Could you check a few things on this model? Use its own coordinates, in mm. Face numbers are marked on the shaded views. Give positions to 0.01 mm unless a question says otherwise; leave off trailing zeros. Loops run counter-clockwise (first coordinate to the right, second up) from the corner with the lowest first, then second, coordinate; pieces in that order, holes last. Notation, with made-up numbers: M -21.5,-38.75 L -2.5,-38.75 A27 ccw -2.5,-3.75 Z; hole C 3,-28.5 d5. An arc over 180 degrees is marked long. Use CSV: the item, a comma, the result in double quotes.
```python
from build123d import *

# Parameters (mm, degrees)
SKETCH2_R           = 0.5
BOSS_EXTRUDE1_DEPTH = 3.5


with BuildPart() as part:
    # Sketch1 → Base-Revolve (revolve)
    with BuildSketch(Plane.XY):
        with BuildLine():
            Line((-3.81, 0.1), (1.69, 0.1))
            Line((1.69, 0.1), (1.69, 0))
            Line((1.69, 0), (3.19, 0))
            ThreePointArc((3.19, 0), (3.897106781, 0.292893219), (4.19, 1))
            Line((4.19, 1), (4.19, 1.21))
            ThreePointArc((4.19, 1.21), (4.049208002, 2.388175538), (3.634760961, 3.5))
            ThreePointArc((3.634760961, 3.5), (4.049208002, 4.611824462), (4.19, 5.79))
            Line((4.19, 5.79), (4.19, 23.2))
            ThreePointArc((4.19, 23.2), (3.604213562, 24.614213562), (2.19, 25.2))
            Line((2.19, 25.2), (1.69, 25.2))
            Line((1.69, 25.2), (1.69, 25.1))
            Line((1.69, 25.1), (-3.81, 25.1))
            Line((-3.81, 25.1), (-3.81, 0.1))
        make_face()
    revolve(axis=Axis((-3.81, 25.2, 0), (0, -1, 0)))

    # Sketch2 → Boss-Extrude1 (add)
    with BuildSketch(Plane.XZ.offset(-0.1)):
        Circle(SKETCH2_R)
        with Locations((-7.62, 0)):
            Circle(SKETCH2_R)
    extrude(amount=BOSS_EXTRUDE1_DEPTH)


solid = part.part
```
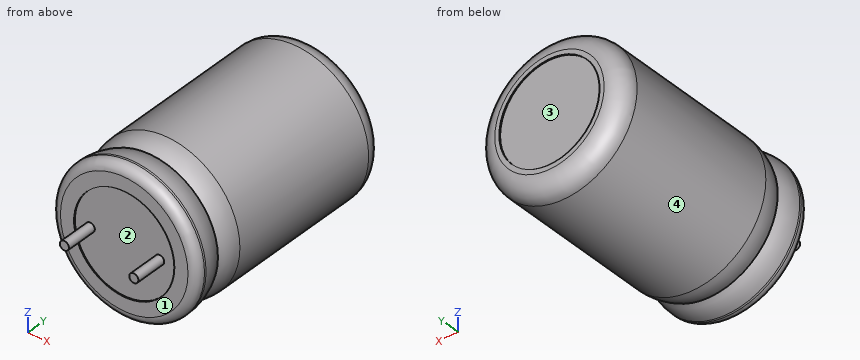
1. I'm going to push flat-ended pins straight in: pin 1 Ø4 at (y, z) = (3.5, 4.5) entering from +X; pin 2 Ø6 at (x, z) = (-2.5, -2) entering from +Y; pin 3 Ø4 at (y, z) = (16, -5.5) entering from +X. Where does each tip first touch, or does it pass through?
Outcome:
pin 1,"x = 3.52"
pin 2,"y = 25.1"
pin 3,"x = 3.38"
2. Please list where these lines run through material, in increasing order: line 1 (Y direction, x = -0.75, z = 3.75); line 2 (X direction, y = -0.25, z = 0.25); line 3 (X direction, y = 18.75, z = -5.25).
Outcome:
line 1,"0.1 to 25.1"
line 2,"-8.05 to -7.19, -0.43 to 0.43"
line 3,"-9.85 to 2.23"
3. I want a section at A-A, the plane y = -1. List the corners of the cut face in (x, z) for me, then the cut area to 3 significant figures.
Outcome:
outline,"C -7.62,0 d1; C 0,0 d1"
area,"1.57 mm2"
4. If we mould it in two halves opening along Z, with no side actions, what happens to the marked faces 1, 2, 3 and 4? For each: +Z half, -Z half, draft (parallel to the pull), parting line (faces both ways), or undercut.
Outcome:
face 1,"draft"
face 2,"undercut"
face 3,"undercut"
face 4,"parting line"
5. I want a section at B-B, the plane y = 9.75. List the corners of the cut face in (x, z) for me, then the cut area to 3 significant figures.
Outcome:
outline,"C -3.81,0 d16"
area,"201 mm2"
